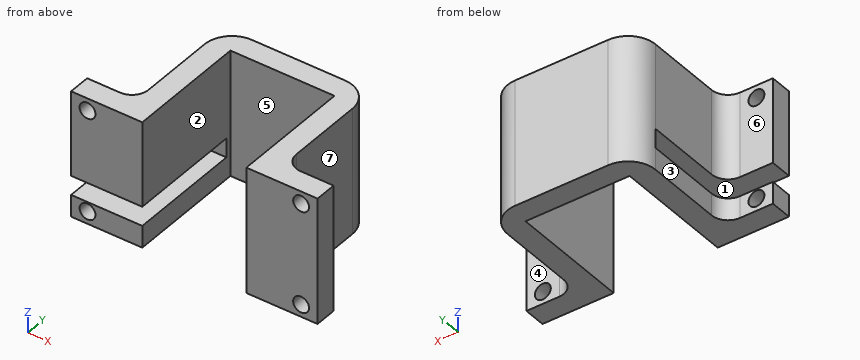
from build123d import *

# Parameters (mm, degrees)
BOSS_EXTRUDE1_DEPTH     = 23
SKETCH3_R               = 1.45
CUT_EXTRUDE1_DEPTH      = 23
CUT_EXTRUDE2_DEPTH      = 23
CUT_EXTRUDE2_DEPTH_BACK = 10
SKETCH4_W               = 3.5
SKETCH4_H               = 21


with BuildPart() as part:
    # Sketch1 → Boss-Extrude1 (new body)
    with BuildSketch(Plane.XY):
        with BuildLine():
            Line((0, 3), (0, 17))
            ThreePointArc((0, 17), (1.464466094, 20.535533906), (5, 22))
            Line((5, 22), (22, 22))
            ThreePointArc((22, 22), (25.535533906, 20.535533906), (27, 17))
            Line((27, 17), (27, 3))
            ThreePointArc((27, 3), (27.878679656, 0.878679656), (30, 0))
            Line((30, 0), (36, 0))
            Line((36, 0), (36, -4))
            Line((36, -4), (23, -4))
            Line((23, -4), (23, 18))
            Line((23, 18), (4, 18))
            Line((4, 18), (4, -4))
            Line((4, -4), (-9, -4))
            Line((-9, -4), (-9, 0))
            Line((-9, 0), (-3, 0))
            ThreePointArc((-3, 0), (-0.878679656, 0.878679656), (0, 3))
        make_face()
    extrude(amount=BOSS_EXTRUDE1_DEPTH)

    # Sketch3 → Cut-Extrude1 (cut)
    with BuildSketch(Plane(origin=(0, 0, 0), x_dir=(1, 0, 0), z_dir=(0, 1, 0))):
        with Locations(Location((-6, -2.25, 0), (0, 0, 270))):
            Circle(SKETCH3_R)
        with Locations(Location((-6, -20.75, 0), (0, 0, 270))):
            Circle(SKETCH3_R)
        with Locations(Location((33, -20.75, 0), (0, 0, 180))):
            Circle(SKETCH3_R)
        with Locations(Location((33, -2.25, 0), (0, 0, 180))):
            Circle(SKETCH3_R)
    extrude(amount=-CUT_EXTRUDE1_DEPTH, mode=Mode.SUBTRACT)

    # Sketch4 → Cut-Extrude2 (cut, two sides: drawn at the far end of the back side and taken through both)
    with BuildSketch(Plane.ZY.offset(-CUT_EXTRUDE2_DEPTH_BACK)):
        with Locations((5.75, 6.5)):
            Rectangle(SKETCH4_W, SKETCH4_H)
    extrude(amount=CUT_EXTRUDE2_DEPTH + CUT_EXTRUDE2_DEPTH_BACK, mode=Mode.SUBTRACT)


solid = part.part
CAD build for the part. Positions are in the model's coordinates, mm. Face numbers are marked on the shaded views. A direction names the side the tool comes from. Round coordinates to 2 decimals unless told otherwise and drop trailing zeros. Write each loop counter-clockwise with the first axis right and the second up, starting at its lowest first coordinate (ties: lowest second). Pieces come first, ordered by that corner, then holes.
(1) Slice it at D-D, the plane z = 2.25. Write the cut outline in (x, y), and give its area (3 significant figures).
(2) 3-axis set-ups, long thin cutter, end or side, ignore diameter. For the marked faces 1, 2, 3 and 4: which of +Z, -Z, +X, -X, +Y, -Y reach the whole face in a straight line?
(3) Drop flat-ended pins along their axis: P1, Ø4.5, axis at x = -6, z = 20.75, coming from the -Y side; P2, Ø4.5, axis at x = -6, z = 1.5, coming from the +Y side; P3, Ø1.5, axis at y = 6, z = 13, coming from the -X side; P4, Ø6.5, axis at y = 9, z = 10, coming from the +X side. Give the stop position or say it passes through.
(4) Mould opens along X. For the marked faces 5, 6 and 7 say: pulls with the +X half, pulls with the -X half, needs draft (parallel to the pull), parting line crosses it, or undercut.
(5) Slice it at C-C, the plane x = -6. Write the cut outline in (y, z), and give its area (3 significant figures).
(6) Slice it at B-B, the plane y = 14.25. Write the cut outline in (x, z).
(7) Slice it at A-A, the plane y = -0.5. Write the cut outline in (x, z), and give its area (3 significant figures).
(8) Probe line 1 along Z through (x, y) = (33, -1.6); line 2 along X through (y, z) = (5.25, 13); line 3 along X through (y, z) = (0.75, 18.5). List the from-to ranges inside material, lowest first.
From the geometry:
1. outline: (-9, -4) - (-7.45, -4) - (-7.45, 0) - (-9, 0) - close; (-4.55, -4) - (4, -4) - (4, 18) - (23, 18) - (23, -4) - (31.55, -4) - (31.55, 0) - (30, 0) arc R3 cw to (27, 3) - (27, 17) arc R5 ccw to (22, 22) - (5, 22) arc R5 ccw to (0, 17) - (0, 3) arc R3 cw to (-3, 0) - (-4.55, 0) - close; (34.45, -4) - (36, -4) - (36, 0) - (34.45, 0) - close
1. area: 326 mm2
2. face 1: -X, -Y
2. face 2: +Z, -Z, -Y
2. face 3: +Z, -Z, -X, +Y
2. face 4: +Z, -Z, +X, +Y
3. P1: stops at y = -4
3. P2: stops at y = 0
3. P3: stops at x = 0
3. P4: stops at x = 27
4. face 5: undercut
4. face 6: needs draft
4. face 7: pulls with the +X half
5. outline: (-4, 0) - (0, 0) - (0, 0.8) - (-4, 0.8) - close; (-4, 3.7) - (0, 3.7) - (0, 4) - (-4, 4) - close; (-4, 7.5) - (0, 7.5) - (0, 19.3) - (-4, 19.3) - close; (-4, 22.2) - (0, 22.2) - (0, 23) - (-4, 23) - close
5. area: 54.8 mm2
6. outline: (0, 0) - (4, 0) - (4, 4) - (0, 4) - close; (0, 7.5) - (4, 7.5) - (4, 23) - (0, 23) - close; (23, 0) - (27, 0) - (27, 23) - (23, 23) - close
7. outline: (-9, 0) - (4, 0) - (4, 4) - (-9, 4) - close; (-9, 7.5) - (4, 7.5) - (4, 23) - (-9, 23) - close; (23, 0) - (36, 0) - (36, 23) - (23, 23) - close; hole circle Ø2.9 at (-6, 2.25); hole circle Ø2.9 at (-6, 20.75); hole circle Ø2.9 at (33, 2.25); hole circle Ø2.9 at (33, 20.75)
7. area: 526 mm2
8. line 1: z = 0 to 0.8, 3.7 to 19.3, 22.2 to 23
8. line 2: x = 0 to 4, 23 to 27
8. line 3: x = -1.02 to 4, 23 to 28.02
